Could you check a few things on this model? Use its own coordinates, in mm. A direction names the side the tool comes from. Give positions to 0.01 mm unless a question says otherwise; leave off trailing zeros. Loops run counter-clockwise (first coordinate to the right, second up) from the corner with the lowest first, then second, coordinate; pieces in that order, holes last. Notation, with made-up numbers: M 50,52 L 76,52 A30 ccw 76,88 Z; hole C 25.25,12.25 d7. An arc over 180 degrees is marked long. Return JSON: item names as keys, results as strings. Group by question number.
1. If we section it at A-A (x = 54): Write out the boundary of the cut face in (y, z), plus the area to 3 significant figures.
2. For pin 1 (4 mm diameter, centred on x = 25.5, y = -25, fed in from -Z); pin 2 (10 mm diameter, centred on x = 9, y = 12.5, fed in from +Z); pin 3 (2 mm diameter, centred on x = 86.5, z = 2.5, fed in from -Y), each with a flat end and sliding along its axis, tell me the tip position at first contact or that it passes through.
3. If we mould it in two halves opening along X, with no side actions, what happens to faces 1 (the cylindrical face through (-12, 0, 1)), 2 (the flat face through (48, 29.5, 1)), 3 (the flat face through (27.2, 21.7, 3))? For each: +X half, -X half, draft (parallel to the pull), parting line (faces both ways), or undercut.
4. If we section it at B-B (y = 22.5): Write out the boundary of the cut face in (x, z), plus the area to 3 significant figures.
5. If we section it at D-D (x = 25): State how many separate pieces and enclosed holes the cut face has, plus the area to 3 significant figures.
6. Please list where these lines run through material, in increasing order: line 1 (X direction, y = -25, z = 3.7); line 2 (X direction, y = 3, z = 2.85); line 3 (Y direction, x = 25.5, z = 1.9).
7. If we section it at C-C (y = 0): Write out the boundary of the cut face in (x, z).
8. For faces 4 (the cylindrical face through (95.839, -12.815, 1.521)), 5 (the flat face through (27, 21, 5.2)), 6 (the cylindrical face through (22.55, -22.3, 1.48)), 7 (the cylindrical face through (64.506, 22.764, 4.085)), 8 (the flat face through (75.065, -11.13, 1.479)), which set-ups out of +Z, -Z, +X, -X, +Y, -Y let a thin tool reach every point of the face, with its end or its side?
```python
from build123d import *

# Parameters (mm, degrees)
SKETCH_R        = 4
PAD_DEPTH       = 3
SKETCH002_R     = 6
PAD001_DEPTH    = 3
SKETCH001_R     = 4
POCKET_DEPTH    = 3
SKETCH003_R     = 1.6
POCKET001_DEPTH = 5.201
FILLET_R        = 10
FILLET001_R     = 10


with BuildPart() as part:
    # Sketch → Pad (new body)
    with BuildSketch(Plane.XY):
        with BuildLine():
            ThreePointArc((0, 12), (-12, 0), (0, -12))
            Line((0, -12), (18.5, -32))
            Line((77.5, -32), (18.5, -32))
            Line((96, -12), (77.5, -32))
            ThreePointArc((96, -12), (108, 0), (96, 12))
            Line((77.5, 29.5), (96, 12))
            Line((18.5, 29.5), (77.5, 29.5))
            Line((18.5, 29.5), (0, 12))
        make_face()
        Circle(SKETCH_R, mode=Mode.SUBTRACT)
        with Locations((96, 0)):
            Circle(SKETCH_R, mode=Mode.SUBTRACT)
        Polygon((66.376801, -20.522703), (84, -1.470596), (84, 1.470596), (66.376801, 18.141189), (29.623199, 18.141189), (12, 1.470596), (12, -1.470596), (29.623199, -20.522703), align=None, mode=Mode.SUBTRACT)
    extrude(amount=PAD_DEPTH)

    # Sketch002 → Pad001 (join)
    with BuildSketch(Plane.XY.offset(2.2)):
        with Locations((25.5, -25)):
            Circle(SKETCH002_R)
        with Locations((70.5, -25)):
            Circle(SKETCH002_R)
        with Locations((25.5, 22.5)):
            Circle(SKETCH002_R)
        with Locations((70.5, 22.5)):
            Circle(SKETCH002_R)
    extrude(amount=PAD001_DEPTH)

    # Sketch001 → Pocket (cut)
    with BuildSketch(Plane.XY):
        with Locations((25.5, -25)):
            Circle(SKETCH001_R)
        with Locations((70.5, -25)):
            Circle(SKETCH001_R)
        with Locations((25.5, 22.5)):
            Circle(SKETCH001_R)
        with Locations((70.5, 22.5)):
            Circle(SKETCH001_R)
    extrude(amount=POCKET_DEPTH, mode=Mode.SUBTRACT)

    # Sketch003 → Pocket001 (cut, through all)
    with BuildSketch(Plane.XY):
        with Locations((25.5, -25)):
            Circle(SKETCH003_R)
        with Locations((70.5, -25)):
            Circle(SKETCH003_R)
        with Locations((25.5, 22.5)):
            Circle(SKETCH003_R)
        with Locations((70.5, 22.5)):
            Circle(SKETCH003_R)
    extrude(amount=POCKET001_DEPTH, mode=Mode.SUBTRACT)

    # Fillet
    fillet_edges = [part.edges().sort_by_distance(p)[0] for p in [
        (77.5, 29.5, 1.5),
        (18.5, 29.5, 1.5),
    ]]
    fillet(fillet_edges, radius=FILLET_R)

    # Fillet001
    fillet001_edges = [part.edges().sort_by_distance(p)[0] for p in [
        (77.5, -32, 1.5),
        (96, -12, 1.5),
    ]]
    fillet(fillet001_edges, radius=FILLET001_R)


solid = part.part
```
Answer:
{
 "1": {"outline": "M -32,0 L -20.52,0 L -20.52,3 L -32,3 Z; M 18.14,0 L 29.5,0 L 29.5,3 L 18.14,3 Z", "area": "68.5 mm²"},
 "2": {"pin 1": "stops at z = 3", "pin 2": "stops at z = 3", "pin 3": "stops at y = -23.35"},
 "3": {"face 1": "-X half", "face 2": "draft", "face 3": "undercut"},
 "4": {"outline": "M 11.1,0 L 21.5,0 L 21.5,3 L 23.9,3 L 23.9,5.2 L 19.5,5.2 L 19.5,3 L 11.1,3 Z; M 27.1,3 L 29.5,3 L 29.5,0 L 66.5,0 L 66.5,3 L 68.9,3 L 68.9,5.2 L 64.5,5.2 L 64.5,3 L 31.5,3 L 31.5,5.2 L 27.1,5.2 Z; M 72.1,3 L 74.5,3 L 74.5,0 L 84.9,0 L 84.9,3 L 76.5,3 L 76.5,5.2 L 72.1,5.2 Z", "area": "212 mm²"},
 "5": {"separate pieces": "4", "enclosed holes": "0", "area": "88.2 mm²"},
 "6": {"line 1": "x = 19.5 to 23.9, 27.1 to 31.5, 64.5 to 68.9, 72.1 to 76.5", "line 2": "x = -11.62 to -2.65, 2.65 to 13.62, 82.38 to 93.35, 98.65 to 107.62", "line 3": "y = -32 to -29, -21 to -16.07, 14.24 to 18.5, 26.5 to 29.5"},
 "7": {"outline": "M -12,0 L -4,0 L -4,3 L -12,3 Z; M 4,0 L 12,0 L 12,3 L 4,3 Z; M 84,0 L 92,0 L 92,3 L 84,3 Z; M 100,0 L 108,0 L 108,3 L 100,3 Z"},
 "8": {"face 4": "+Z, -Z, +X, -Y", "face 5": "+Z, +X, -X, +Y, -Y", "face 6": "-Z", "face 7": "+Z", "face 8": "+Z, -Z"}
}
